Geometry check sheet. Reference: the model listing, model coordinates, mm. Round coordinates to 2 decimals unless told otherwise and drop trailing zeros. Write each loop counter-clockwise with the first axis right and the second up, starting at its lowest first coordinate (ties: lowest second). Pieces come first, ordered by that corner, then holes. Notation, with made-up numbers: (15, 47.5) - (58, 47.5) arc R26 cw to (58, 67.5) - close; hole circle Ø9 at (51, -39.5). An arc over 180 degrees is marked (long way). One line per question, with ' | ' between items. Start each with the question number.
from build123d import *

# Parameters (mm, degrees)
F0_W     = 40.16
F0_H     = 13.47
F0_W_2   = 3.5
F0_H_2   = 1
F0_R     = 1.5
F0_W_3   = 5.5
F0_H_3   = 5.5
F1_DEPTH = 1
F2_DEPTH = 1.8
F3_DEPTH = 2
F4_R     = 0.99999
F5_R     = 0.9
F6_DEPTH = 0.5
F7_W     = 3
F7_H     = 8.5
F8_DEPTH = 1.2


# Not quite as in the source:
# - a fillet or chamfer is up to 0.001 mm smaller than in the source, because OpenCascade refuses the exact size


with BuildPart() as f1:
    # F0 (on Top) → F1 (new body)
    with BuildSketch(Plane.XY):
        with Locations((1.9053274065, 3.3154582972)):
            Rectangle(F0_W, F0_H)
        with Locations((-9.2646725935, -1.7195417028)):
            Rectangle(F0_W_2, F0_H_2, mode=Mode.SUBTRACT)
        with Locations((-2.7646725935, -1.7195417028)):
            Rectangle(F0_W_2, F0_H_2, mode=Mode.SUBTRACT)
        with Locations((3.7353274065, -1.7195417028)):
            Rectangle(F0_W_2, F0_H_2, mode=Mode.SUBTRACT)
        with Locations((10.2353274065, -1.7195417028)):
            Rectangle(F0_W_2, F0_H_2, mode=Mode.SUBTRACT)
        with Locations((19.4853274065, -1.1195417028)):
            Circle(F0_R, mode=Mode.SUBTRACT)
        with Locations((-15.6746725935, 7.7504582972)):
            Circle(F0_R, mode=Mode.SUBTRACT)
        with Locations((18.4353274065, 6.3004582972)):
            Rectangle(F0_W_3, F0_H_3, mode=Mode.SUBTRACT)
        with Locations((-9.2646725935, -1.7195417028)):
            Rectangle(F0_W_2, F0_H_2)
        with Locations((-2.7646725935, -1.7195417028)):
            Rectangle(F0_W_2, F0_H_2)
        with Locations((3.7353274065, -1.7195417028)):
            Rectangle(F0_W_2, F0_H_2)
        with Locations((10.2353274065, -1.7195417028)):
            Rectangle(F0_W_2, F0_H_2)
        with Locations((18.4353274065, 6.3004582972)):
            Rectangle(F0_W_3, F0_H_3)
    extrude(amount=F1_DEPTH)

    # F0 (on Top) → F2 (join)
    with BuildSketch(Plane.XY):
        with Locations((-9.2646725935, -1.7195417028)):
            Rectangle(F0_W_2, F0_H_2)
        with Locations((-2.7646725935, -1.7195417028)):
            Rectangle(F0_W_2, F0_H_2)
        with Locations((3.7353274065, -1.7195417028)):
            Rectangle(F0_W_2, F0_H_2)
        with Locations((10.2353274065, -1.7195417028)):
            Rectangle(F0_W_2, F0_H_2)
    extrude(amount=F2_DEPTH)

    # F0 (on Top) → F3 (join)
    with BuildSketch(Plane.XY):
        with Locations((18.4353274065, 6.3004582972)):
            Rectangle(F0_W_3, F0_H_3)
    extrude(amount=F3_DEPTH)

    # F4 (radius 1 in the source; OpenCascade refuses exactly that, so slightly less here)
    f4_edges = [f1.edges().sort_by_distance(p)[0] for p in [
        (21.185327, 6.300458, 2),
        (15.685327, 6.300458, 2),
        (18.435327, 3.550458, 2),
        (18.435327, 9.050458, 2),
    ]]
    fillet(f4_edges, radius=F4_R)

    # F5 (on face) → F6 (join)
    with BuildSketch(Plane.XY.offset(2)):
        with Locations((18.4353274065, 6.3004582972)):
            Circle(F5_R)
    extrude(amount=F6_DEPTH)

    # F7 (on face) → F8 (join)
    with BuildSketch(Plane(origin=(0, 0, 0), x_dir=(1, 0, 0), z_dir=(0, 0, -1))):
        with Locations((-1.5146725935, -4.8004582972)):
            Rectangle(F7_W, F7_H)
    extrude(amount=F8_DEPTH)


solid = f1.part
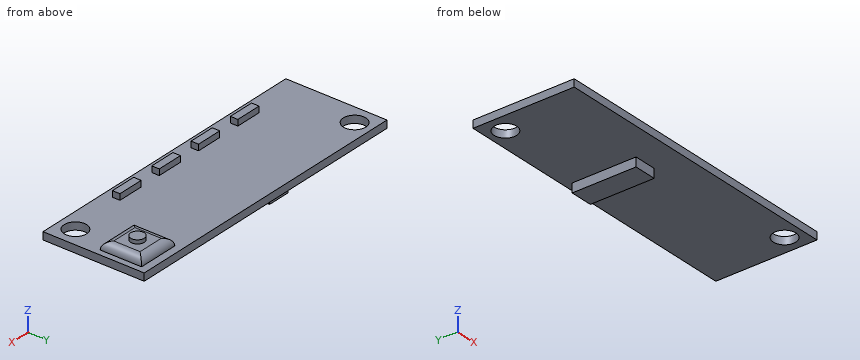
Q1. Thickness scan on line 1 (X direction, y = 6.75, z = -0.95); line 2 (Z direction, x = 14, y = 2.5); line 3 (X direction, y = -1.25, z = 0.45). Record the ranges inside material, lowest first.
Q2. Go/stop test with flat-tipped pins: P1, Ø5, axis at x = -8, y = 0, coming from the -Z side; P2, Ø3, axis at x = 12.5, y = 7.5, coming from the +Z side; P3, Ø0.6, axis at x = 4, z = 1.5, coming from the -Y side. Record where each tip stops, or that it passes through.
Q3. Section check A-A, the plane x = -4. Record the cut outline in (y, z).
Q4. Section check B-B, the plane y = 2.5. Record the cut outline in (x, z).
Q5. Section check C-C, the plane z = 0.45. Record the cut outline in (x, y), then the cut area to 3 significant figures.
Result sheet:
1) line 1: -3.01 to -0.01 | line 2: 0 to 1 | line 3: -18.17 to 17.99, 20.98 to 21.99
2) P1: z = 0 | P2: z = 1 | P3: y = -2.22
3) outline: (-3.42, 0) - (10.05, 0) - (10.05, 1) - (-1.22, 1) - (-1.22, 1.8) - (-2.22, 1.8) - (-2.22, 1) - (-3.42, 1) - close
4) outline: (-18.17, 0) - (-3.01, 0) - (-3.01, -1.2) - (-0.01, -1.2) - (-0.01, 0) - (21.99, 0) - (21.99, 1) - (-18.17, 1) - close
5) outline: (-18.17, -3.42) - (21.99, -3.42) - (21.99, 10.05) - (-18.17, 10.05) - close; hole circle Ø3 at (-15.67, 7.75); hole circle Ø3 at (19.49, -1.12) | area: 527 mm²
